from build123d import *

# Parameters (mm, degrees)
BOSS_EXTRU_1_DEPTH      = 18
BOSS_EXTRU_1_DEPTH_BACK = 30
ESQUISSE2_R             = 7.5
CHANFREIN1_SIZE         = 2
ESQUISSE3_R             = 4.5
BOSS_EXTRU_2_DEPTH      = 15
CHANFREIN2_SIZE         = 1
ESQUISSE4_R             = 3.5
BOSS_EXTRU_3_DEPTH      = 10
BOSS_EXTRU_4_DEPTH      = 5


with BuildPart() as part:
    # Esquisse1 → Révolution1 (revolve)
    with BuildSketch(Plane.XY, mode=Mode.PRIVATE) as r_volution1_sk:
        Polygon((-12, 0), (-14, 0), (-14, 12), (-3, 12), (-3, 18), (0, 18), (0, 0), (-10, 0), (-10, 10), (-12, 10), align=None)
    revolve(r_volution1_sk.sketch.rotate(Axis((0, 0, 0), (0, 1, 0)), 270), axis=Axis((0, 0, 0), (0, 1, 0)))

    # Esquisse2 → Boss.-Extru.1 (add, two sides: drawn at the far end of the back side and taken through both)
    with BuildSketch(Plane.XY.offset(-BOSS_EXTRU_1_DEPTH_BACK)):
        with Locations((0, 22)):
            Circle(ESQUISSE2_R)
    extrude(amount=BOSS_EXTRU_1_DEPTH + BOSS_EXTRU_1_DEPTH_BACK)

    # Chanfrein1
    chanfrein1_edges = [part.edges().sort_by_distance(p)[0] for p in [
        (-7.5, 22, -30),
        (-7.5, 22, 18),
    ]]
    chamfer(chanfrein1_edges, length=CHANFREIN1_SIZE)

    # Esquisse3 → Boss.-Extru.2 (add)
    with BuildSketch(Plane.XY.offset(18)):
        with Locations((0, 22)):
            Circle(ESQUISSE3_R)
    extrude(amount=BOSS_EXTRU_2_DEPTH)

    # Chanfrein2
    chanfrein2_edges = [part.edges().sort_by_distance(p)[0] for p in [
        (-4.5, 22, 33),
    ]]
    chamfer(chanfrein2_edges, length=CHANFREIN2_SIZE)

    # Esquisse4 → Boss.-Extru.3 (add)
    with BuildSketch(Plane(origin=(0, 0, -30), x_dir=(-1, 0, 0), z_dir=(0, 0, -1))):
        with Locations((0, 22)):
            Circle(ESQUISSE4_R)
    extrude(amount=BOSS_EXTRU_3_DEPTH)

    # Esquisse5 → Boss.-Extru.4 (add)
    with BuildSketch(Plane(origin=(0, 0, -40), x_dir=(-1, 0, 0), z_dir=(0, 0, -1))):
        with BuildLine():
            Line((-2, 28.92820323), (-2, 32.6))
            ThreePointArc((-2, 32.6), (-1.443502884, 33.943502884), (-0.1, 34.5))
            Line((-0.1, 34.5), (0.1, 34.5))
            ThreePointArc((0.1, 34.5), (1.443502884, 33.943502884), (2, 32.6))
            Line((2, 32.6), (2, 28.92820323))
            ThreePointArc((2, 28.92820323), (3.339745962, 23.92820323), (7, 20.267949192))
            Line((7, 20.267949192), (10.17986928, 18.432050808))
            ThreePointArc((10.17986928, 18.432050808), (11.06512835, 17.278358726), (10.875317547, 15.83660254))
            Line((10.875317547, 15.83660254), (10.775317547, 15.66339746))
            ThreePointArc((10.775317547, 15.66339746), (9.621625466, 14.77813839), (8.17986928, 14.967949192))
            Line((8.17986928, 14.967949192), (5, 16.803847577))
            ThreePointArc((5, 16.803847577), (0, 18.143593539), (-5, 16.803847577))
            Line((-5, 16.803847577), (-8.17986928, 14.967949192))
            ThreePointArc((-8.17986928, 14.967949192), (-9.621625466, 14.77813839), (-10.775317547, 15.66339746))
            Line((-10.775317547, 15.66339746), (-10.875317547, 15.83660254))
            ThreePointArc((-10.875317547, 15.83660254), (-11.06512835, 17.278358726), (-10.17986928, 18.432050808))
            Line((-10.17986928, 18.432050808), (-7, 20.267949192))
            ThreePointArc((-7, 20.267949192), (-3.339745962, 23.92820323), (-2, 28.92820323))
        make_face()
    extrude(amount=BOSS_EXTRU_4_DEPTH)


solid = part.part
Can you work these out from the model? Positions are in its coordinate system, mm. A direction names the side the tool comes from. Round coordinates to 2 decimals unless told otherwise and drop trailing zeros. Write each loop counter-clockwise with the first axis right and the second up, starting at its lowest first coordinate (ties: lowest second). Pieces come first, ordered by that corner, then holes. Notation, with made-up numbers: (-37, 20) -> (-21, 20) arc R16 ccw to (-21, 51) -> close; hole circle Ø2 at (45, 54). An arc over 180 degrees is marked (long way). Use one line per item in the form item = value. Start each with the question number.
Q1. Imagine slicing it at B-B (y = 22). Please give me the cut outline in (x, z).
Q2. We'd pull the mould along Z, two halves only. Please class faces 5 (the face through (-9, 10, -5)), 6 (the face through (-0.59, 26.46, 24.9)), 7 (the face through (0.46, 25.47, -34.93)), 8 (the face through (-5, 22, 18)): +Z half, -Z half, draft (parallel to the pull), parting line (faces both ways), or undercut.
Q3. Imagine slicing it at A-A (z = 0). Please give me the cut outline in (x, y).
Q4. I'm going to push flat-ended pins straight in: P1, Ø4, axis at x = 2, z = 23, coming from the +Y side; P2, Ø6, axis at x = -6, z = -2.5, coming from the +Y side; P3, Ø7, axis at x = 6, z = 1, coming from the -Y side; P4, Ø12, axis at x = -9.5, y = 8, coming from the +Z side. Where does each tip first touch, or does it pass through?
Q5. Imagine slicing it at C-C (z = 15). Please give me the cut outline in (x, y).
Q6. If I drill on probe 1 along X at (y, z) = (7.75, 0); probe 2 along Z at (x, y) = (-5.5, 4), over which ranges is the centre line in solid material (lowest first)? Write a range as [from, to].
Q7. Which directions (+Z, -Z, +X, -X, +Y, -Y) give clear straight access to the entire face, cutting with the end or side of a thin tool? Please do faces 1 (the face through (3.38, 23.86, -42.46)), 2 (the face through (9.76, 5.07, 2.17)), 3 (the face through (4, 22, -30)), 4 (the face through (-0.073, 18.143, -42.465)).
Q8. Imagine slicing it at D-D (y = 13). Please give me the cut outline in (x, z).
Worked out:
q1.outline = (-7.5, -28) -> (-5.5, -30) -> (-3.5, -30) -> (-3.5, -40) -> (-4.79, -40) -> (-4.79, -45) -> (4.79, -45) -> (4.79, -40) -> (3.5, -40) -> (3.5, -30) -> (5.5, -30) -> (7.5, -28) -> (7.5, 16) -> (5.5, 18) -> (4.5, 18) -> (4.5, 32) -> (3.5, 33) -> (-3.5, 33) -> (-4.5, 32) -> (-4.5, 18) -> (-5.5, 18) -> (-7.5, 16) -> close
q2.face_5 = undercut
q2.face_6 = draft
q2.face_7 = undercut
q2.face_8 = +Z half
q3.outline = (-14, 0) -> (-12, 0) -> (-12, 10) -> (-10, 10) -> (-10, 0) -> (10, 0) -> (10, 10) -> (12, 10) -> (12, 0) -> (14, 0) -> (14, 12) -> (3, 12) -> (3, 15.13) arc R7.5 ccw (long way) to (-3, 15.13) -> (-3, 12) -> (-14, 12) -> close
q4.P1 = 26.5
q4.P2 = 28.87
q4.P3 = 0
q4.P4 = 13.56
q5.outline = circle Ø15 at (0, 22)
q6.probe_1 = [-14, -12], [-10, 10], [12, 14]
q6.probe_2 = [-12.87, -10.67], [-8.35, 8.35], [10.67, 12.87]
q7.face_1 = -Z, +X, +Y
q7.face_2 = -Y
q7.face_3 = none
q7.face_4 = -Z, -Y
q8.outline = circle Ø6 at (0, 0)
